Here's how the part is built. I have some questions about the finished solid (model axes, mm). Give positions to 0.01 mm unless a question says otherwise; leave off trailing zeros. Loops run counter-clockwise (first coordinate to the right, second up) from the corner with the lowest first, then second, coordinate; pieces in that order, holes last. Notation, with made-up numbers: (28, -3.5) - (84, -3.5) arc R18 ccw to (84, 7.5) - close; hole circle Ø1 at (14, -14.75). An arc over 180 degrees is marked (long way). Return JSON: item names as keys, results as strings. Group by question number.
(1) If we section it at A-A (z = -4): Please give me the cut outline in (x, y).
(2) For P1, Ø4, axis at x = 44, y = 18, coming from the -Z side, with a flat end and sliding along its axis, tell me the tip position at first contact or that it passes through.
(3) If we section it at B-B (x = 44): State how many separate pieces and enclosed holes the cut face has, then the cut area to 3 significant figures.
(4) I need wall thicknesses on probe 1 along Y at (x, z) = (44, -3); probe 2 along Y at (x, z) = (44, -2.05); probe 3 along Z at (x, y) = (47, 26). Which ranges of each line are inside material? Lowest first, please. Write a range as [from, to].
(5) If we section it at C-C (z = -1): Please give me the cut outline in (x, y).
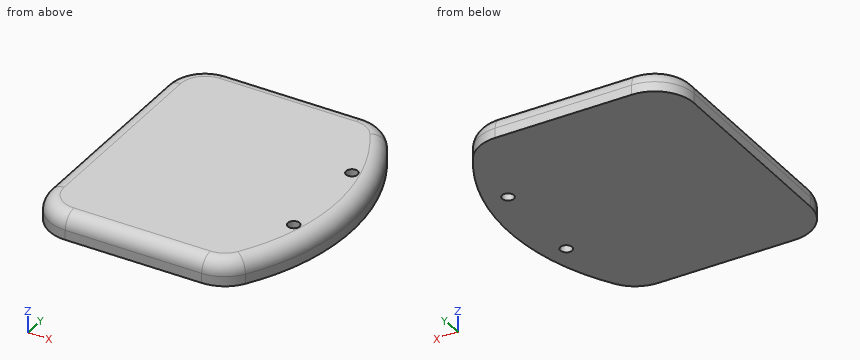
```python
from build123d import *

# Parameters (mm, degrees)
EXTRUDE_1_DEPTH       = 5
FILLET_3_R            = 8
FILLET_4_R            = 3
HOLE_WIZARD_M32_D     = 2.4
HOLE_WIZARD_M32_DEPTH = 9.278967257
HOLE_WIZARD_M32_TIP   = 0.721032743


with BuildPart() as part:
    # Эскиз1 → Бобышка-Вытянуть1 (new body)
    with BuildSketch(Plane.XY):
        with BuildLine():
            Line((0, 0), (40, 0))
            ThreePointArc((40, 0), (49.772170092, 28), (40, 56))
            Line((40, 56), (0, 56))
            Line((0, 56), (0, 0))
        make_face()
    extrude(amount=-EXTRUDE_1_DEPTH)

    # Скругление3
    fillet_3_edges = [part.edges().sort_by_distance(p)[0] for p in [
        (0, 0, -2.5),
        (0, 56, -2.5),
        (40, 56, -2.5),
        (40, 0, -2.5),
    ]]
    fillet(fillet_3_edges, radius=FILLET_3_R)

    # Скругление4
    fillet_4_edges = [part.edges().sort_by_distance(p)[0] for p in [
        (49.772170092, 28, 0),
        (21.950467462, 0, 0),
        (21.950467462, 56, 0),
        (0, 28, 0),
        (2.343145751, 53.656854249, 0),
        (2.343145751, 2.343145751, 0),
        (39.735345271, 0.978796592, 0),
        (39.735345271, 55.021203408, 0),
    ]]
    fillet(fillet_4_edges, radius=FILLET_4_R)

    # Отверстие с зазором M32
    with Locations(Plane.XY):
        with Locations((44, 38), (44, 18)):
            Hole(HOLE_WIZARD_M32_D / 2, depth=HOLE_WIZARD_M32_DEPTH)
            with Locations((0, 0, -(HOLE_WIZARD_M32_DEPTH + HOLE_WIZARD_M32_TIP / 2))):  # 118° drill point
                Cone(0, HOLE_WIZARD_M32_D / 2, HOLE_WIZARD_M32_TIP, mode=Mode.SUBTRACT)


solid = part.part
```
Values:
{
 "1": {"outline": "(0, 8) arc R8 ccw to (8, 0) - (35.9, 0) arc R8 ccw to (42.63, 3.68) arc R45 ccw to (42.63, 52.32) arc R8 ccw to (35.9, 56) - (8, 56) arc R8 ccw to (0, 48) - close; hole circle Ø2.4 at (44, 18); hole circle Ø2.4 at (44, 38)"},
 "2": {"P1": "z = -5"},
 "3": {"separate pieces": "3", "enclosed holes": "0", "area": "188 mm2"},
 "4": {"probe 1": "[5.95, 16.8], [19.2, 36.8], [39.2, 50.05]", "probe 2": "[6.27, 16.8], [19.2, 36.8], [39.2, 49.73]", "probe 3": "[-5, -0.01]"},
 "5": {"outline": "(0.76, 8) arc R7.24 ccw to (8, 0.76) - (35.9, 0.76) arc R7.24 ccw to (41.99, 4.09) arc R44.24 ccw to (41.99, 51.91) arc R7.24 ccw to (35.9, 55.24) - (8, 55.24) arc R7.24 ccw to (0.76, 48) - close; hole circle Ø2.4 at (44, 18); hole circle Ø2.4 at (44, 38)"}
}
